For this review, take the finished solid that the model builds, in its own axes (mm). A direction names the side the tool comes from. Round coordinates to 2 decimals unless told otherwise and drop trailing zeros. Write each loop counter-clockwise with the first axis right and the second up, starting at its lowest first coordinate (ties: lowest second). Pieces come first, ordered by that corner, then holes.
from build123d import *

# Parameters (mm, degrees)
CROQUIS1_R              = 1.905
CROQUIS1_R_2            = 21.717
SALIENTE_EXTRUIR1_DEPTH = 4.318
CROQUIS1_3_R            = 21.717
CROQUIS1_3_R_2          = 10.541
SALIENTE_EXTRUIR2_DEPTH = 8.636
CROQUIS1_4_R            = 10.541
SALIENTE_EXTRUIR3_DEPTH = 25.908
TALADRO1_D              = 8.636
TALADRO1_DEPTH          = 21.59
CROQUIS5_R              = 4.699
SALIENTE_EXTRUIR4_DEPTH = 10.668
MATRIZC1_COUNT          = 4


with BuildPart() as part:
    # Croquis1 → Saliente-Extruir1 (new body)
    with BuildSketch(Plane(origin=(0, 0, 0), x_dir=(1, 0, 0), z_dir=(0, 1, 0))):
        with BuildLine():
            Line((-36.83, 0), (-42.579167494, -4.33230845))
            ThreePointArc((-42.579167494, -4.33230845), (0, -42.799), (42.579167494, -4.33230845))
            Line((42.579167494, -4.33230845), (36.83, 0))
            Line((36.83, 0), (42.579167494, 4.33230845))
            ThreePointArc((42.579167494, 4.33230845), (0, 42.799), (-42.579167494, 4.33230845))
            Line((-42.579167494, 4.33230845), (-36.83, 0))
        make_face()
        with Locations((32.385, 0)):
            Circle(CROQUIS1_R, mode=Mode.SUBTRACT)
        with Locations((28.046232702, 16.1925)):
            Circle(CROQUIS1_R, mode=Mode.SUBTRACT)
        with Locations((16.1925, 28.046232702)):
            Circle(CROQUIS1_R, mode=Mode.SUBTRACT)
        with Locations((0, 32.385)):
            Circle(CROQUIS1_R, mode=Mode.SUBTRACT)
        with Locations((-16.1925, 28.046232702)):
            Circle(CROQUIS1_R, mode=Mode.SUBTRACT)
        with Locations((-28.046232702, 16.1925)):
            Circle(CROQUIS1_R, mode=Mode.SUBTRACT)
        with Locations((-32.385, 0)):
            Circle(CROQUIS1_R, mode=Mode.SUBTRACT)
        with Locations((-28.046232702, -16.1925)):
            Circle(CROQUIS1_R, mode=Mode.SUBTRACT)
        with Locations((-16.1925, -28.046232702)):
            Circle(CROQUIS1_R, mode=Mode.SUBTRACT)
        with Locations((0, -32.385)):
            Circle(CROQUIS1_R, mode=Mode.SUBTRACT)
        with Locations((16.1925, -28.046232702)):
            Circle(CROQUIS1_R, mode=Mode.SUBTRACT)
        with Locations((28.046232702, -16.1925)):
            Circle(CROQUIS1_R, mode=Mode.SUBTRACT)
        Circle(CROQUIS1_R_2, mode=Mode.SUBTRACT)
    extrude(amount=SALIENTE_EXTRUIR1_DEPTH)

    # Croquis1<3> → Saliente-Extruir2 (add)
    with BuildSketch(Plane(origin=(0, 0, 0), x_dir=(1, 0, 0), z_dir=(0, 1, 0))):
        Circle(CROQUIS1_3_R)
        Circle(CROQUIS1_3_R_2, mode=Mode.SUBTRACT)
    extrude(amount=SALIENTE_EXTRUIR2_DEPTH)

    # Croquis1<4> → Saliente-Extruir3 (add)
    with BuildSketch(Plane(origin=(0, 0, 0), x_dir=(1, 0, 0), z_dir=(0, 1, 0))):
        Circle(CROQUIS1_4_R)
    extrude(amount=SALIENTE_EXTRUIR3_DEPTH)

    # Taladro1
    with Locations(Plane(origin=(0, 25.908, 0), x_dir=(1, 0, 0), z_dir=(0, 1, 0))):
        with Locations((0, 0)):
            Hole(TALADRO1_D / 2, depth=TALADRO1_DEPTH)

    # Croquis5 → Saliente-Extruir4 (add)
    with BuildSketch(Plane.XZ):
        with Locations((28.046232702, -16.1925)):
            Circle(CROQUIS5_R)
    saliente_extruir4 = extrude(amount=SALIENTE_EXTRUIR4_DEPTH)

    # MatrizC1: Saliente-Extruir4 ×4 about axis
    matrizc1_axis = Axis((-0.295191575, 0, 0.170428935), (0, 1, 0))
    for i in range(1, MATRIZC1_COUNT):
        add(saliente_extruir4.rotate(matrizc1_axis, i * 360 / MATRIZC1_COUNT))


solid = part.part
(1) For faces 4 (the face through (-39.664, 2.129, 2.136)), 5 (the face through (0.88, 2.13, -42.79)), 6 (the face through (39.664, 2.129, -2.136)), 7 (the face through (16, 0, 28)), 8 (the face through (-13.48, -5.26, -24.71)), list the 3-axis set-ups (+Z, -Z, +X, -X, +Y, -Y) from which the entire face can be reached by the end or side of a thin tool; tool diameter is ignored.
Geometry check:
face 4: -X, +Y, -Y
face 5: -Z, +Y, -Y
face 6: +X, +Y, -Y
face 7: +Y
face 8: -Y
(2) For line 1 along Y through (x, z) = (-11, -27.5); line 2 along Y through (x, z) = (13.5, 3); line 3 along X through (y, z) = (3, 33), list the stretches that pass through material, from the lowest coordinate up.
Geometry check:
line 1: y = 0 to 4.32
line 2: y = 0 to 8.64
line 3: x = -27.25 to -1.8, 1.8 to 27.25
(3) We need section B-B, the plane y = 17. Give the boundary of the cut face in (x, z), and give its area (3 significant figures).
Geometry check:
outline: circle Ø21.08 at (0, 0); hole circle Ø8.64 at (0, 0)
area: 290 mm2
(4) For pin 1 Ø1.5 at (x, y) = (7, 11) entering from -Z; pin 2 Ø3 at (x, z) = (-28.05, -16.19) entering from +Y; pin 3 Ø1.9 at (x, z) = (16, 28) entering from +Y; pin 4 Ø4.5 at (x, z) = (-32.385, 0) entering from +Y, all flat-tipped, find the tip position at first contact; note any pin that passes through.
Geometry check:
pin 1: stops at z = -8.49
pin 2: passes through
pin 3: stops at y = 0
pin 4: stops at y = 4.32
(5) Mouldability with a two-part tool opening along Z and no side actions: class faces 1 (the face through (27.435, -5.259, -11.533)), 2 (the face through (29.806, 2.129, 16.922)), 3 (the face through (-17, -10.668, -28)) as pulls with the +Z half, pulls with the -Z half, needs draft (parallel to the pull), parting line crosses it, or undercut.
Geometry check:
face 1: parting line crosses it
face 2: undercut
face 3: needs draft
(6) We need section C-C, the plane y = -8. Give the boundary of the cut face in (x, z).
Geometry check:
outline: circle Ø9.4 at (-28.64, 16.53); circle Ø9.4 at (-16.66, -28.17); circle Ø9.4 at (16.07, 28.51); circle Ø9.4 at (28.05, -16.19)
(7) We need section A-A, the plane x = 0. Give the boundary of the cut face in (y, z), and give its area (3 significant figures).
Geometry check:
outline: (0, -42.8) - (4.32, -42.8) - (4.32, -34.29) - (0, -34.29) - close; (0, -30.48) - (4.32, -30.48) - (4.32, -21.72) - (8.64, -21.72) - (8.64, -10.54) - (25.91, -10.54) - (25.91, -4.32) - (4.32, -4.32) - (4.32, 4.32) - (25.91, 4.32) - (25.91, 10.54) - (8.64, 10.54) - (8.64, 21.72) - (4.32, 21.72) - (4.32, 30.48) - (0, 30.48) - close; (0, 34.29) - (4.32, 34.29) - (4.32, 42.8) - (0, 42.8) - close
area: 702 mm2
